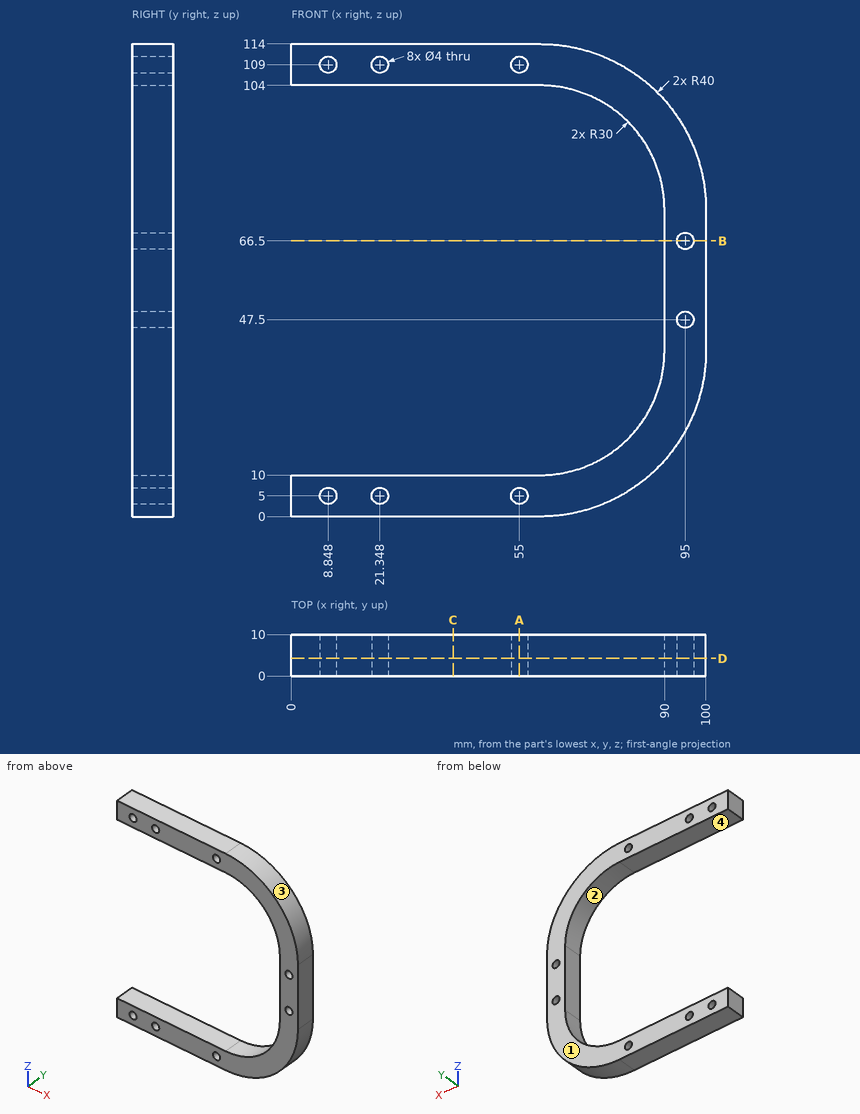
Input: dimensioned drawing with shaded views. Units: mm. Origin: part minimum x, y, z. Give positions to 0.01 mm unless a question says otherwise; leave off trailing zeros. Order: outer loops, then holes, each group sorted by start corner. A loop starts at its lowest first (then second) coordinate and runs counter-clockwise, first axis right, second up.
(1) Section query C-C (x = 39). Return the cut outline in (y, z), plus the area to 3 significant figures.
(2) Material intervals for line 1 along Z through (x, y) = (38, 2); line 2 along Z through (x, y) = (56.5, 6.25) (1 decimal); line 3 along X through (y, z) = (2, 55.5), sorted ascending.
(3) Contact query for flat-ended pins moving along their axis: P1, Ø2, axis at y = 5.5, z = 37, coming from the +X side; P2, Ø3.5, axis at x = 8.85, z = 109, coming from the -Y side; P3, Ø5, axis at y = 5.5, z = 59.5, coming from the -X side; P4, Ø3, axis at y = 5.5, z = 81, coming from the +X side. Output: stop coordinate, or through.
(4) Section query B-B (z = 66.5). Return the cut outline in (x, y).
(5) Section query D-D (y = 4.25). State how many separate pieces and enclosed holes the cut face has, plus the area to 3 significant figures.
(6) Pull-direction query (Z, two-part tool) for the marked faces 1, 2, 3 and 4; classes: +Z half, -Z half, draft (parallel to the pull), parting line (faces both ways), or undercut.
(7) Section query A-A (x = 55). Return the cut outline in (y, z), plus the area to 3 significant figures.
Outcome:
1. outline: (0, 0) - (10, 0) - (10, 10) - (0, 10) - close; (0, 104) - (10, 104) - (10, 114) - (0, 114) - close
1. area: 200 mm2
2. line 1: z = 0 to 10, 104 to 114
2. line 2: z = 0 to 3.7, 6.3 to 10, 104 to 107.7, 110.3 to 114
2. line 3: x = 90 to 100
3. P1: stops at x = 99.95
3. P2: passes through
3. P3: stops at x = 90
3. P4: stops at x = 99.62
4. outline: (90, 0) - (93, 0) - (93, 10) - (90, 10) - close; (97, 0) - (100, 0) - (100, 10) - (97, 10) - close
5. separate pieces: 1
5. enclosed holes: 8
5. area: 2,540 mm2
6. face 1: draft
6. face 2: undercut
6. face 3: +Z half
6. face 4: undercut
7. outline: (0, 0) - (10, 0) - (10, 3) - (0, 3) - close; (0, 7) - (10, 7) - (10, 10) - (0, 10) - close; (0, 104) - (10, 104) - (10, 107) - (0, 107) - close; (0, 111) - (10, 111) - (10, 114) - (0, 114) - close
7. area: 120 mm2
